from build123d import *

# Parameters (mm, degrees)
EXTRUDE_THIN1_DEPTH      = 28
EXTRUDE_THIN1_DEPTH_BACK = 8


with BuildPart() as part:
    # Sketch1 → Extrude-Thin1 (new, two sides: drawn at the far end of the back side and taken through both)
    with BuildSketch(Plane.XY.offset(-EXTRUDE_THIN1_DEPTH_BACK)):
        with BuildLine():
            Line((19.383566169, -68.309294305), (57.022380557, -25.814786092))
            ThreePointArc((57.022380557, -25.814786092), (65.70728891, -19.214238602), (76.255341013, -16.4333292))
            Line((76.255341013, -16.4333292), (228.091165061, -7.048771065))
            ThreePointArc((228.091165061, -7.048771065), (323.514042398, -112.549255422), (199.474713255, -182.192076622))
            Line((199.474713255, -182.192076622), (-76.082369589, -70.323577063))
            ThreePointArc((-76.082369589, -70.323577063), (-86.509762237, -25.814215154), (-41.067256055, -30.793416585))
            Line((-41.067256055, -30.793416585), (-22.813516306, -63.686280276))
            ThreePointArc((-22.813516306, -63.686280276), (-2.911096467, -76.915520396), (19.383566169, -68.309294305))
        make_face()
        with BuildLine():
            Line((26.869376151, -74.939727844), (64.508190539, -32.44521963))
            ThreePointArc((64.508190539, -32.44521963), (70.091345909, -28.20201053), (76.872236546, -26.414283057))
            Line((76.872236546, -26.414283057), (228.708060595, -17.029724922))
            ThreePointArc((228.708060595, -17.029724922), (313.644907456, -110.93674946), (203.236273822, -172.926513385))
            Line((203.236273822, -172.926513385), (-72.320809021, -61.058013827))
            ThreePointArc((-72.320809021, -61.058013827), (-79.024132867, -32.444852599), (-49.811093178, -35.645767804))
            Line((-49.811093178, -35.645767804), (-31.557353429, -68.538631496))
            ThreePointArc((-31.557353429, -68.538631496), (-4.00015673, -86.856040893), (26.869376151, -74.939727844))
        make_face(mode=Mode.SUBTRACT)
    extrude(amount=EXTRUDE_THIN1_DEPTH + EXTRUDE_THIN1_DEPTH_BACK)


solid = part.part
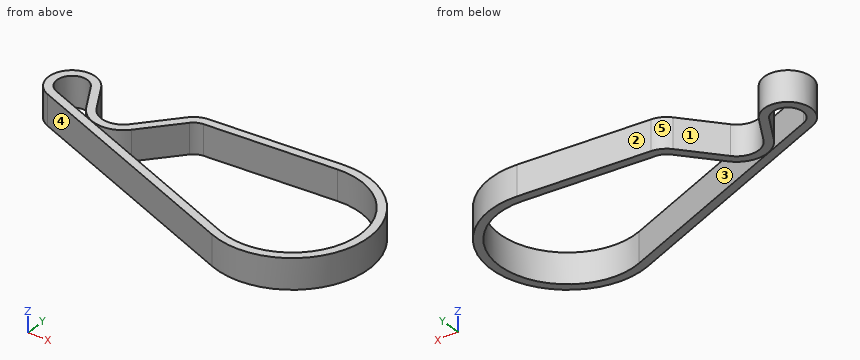
Read the model definition and answer for the solid it produces. Units are mm, in the model's axes. Face numbers are marked on the shaded views. A direction names the side the tool comes from. Round coordinates to 2 decimals unless told otherwise and drop trailing zeros. Loops run counter-clockwise (first coordinate to the right, second up) from the corner with the lowest first, then second, coordinate; pieces in that order, holes last.
Q1. Section C-C on y = -44.38 is taken. Write down the section's boundary in (x, z), and give its area (3 significant figures).
Q2. Section A-A on z = 2.5 is taken. Write down the section's boundary in (x, y).
Q3. Determine the mould class of the marked faces 1 and 2 for opening direction X: released by +X, released by -X, zero draft, split by the parting line, or undercut.
Q4. Consider probe 1 along X at (y, z) = (-70, -4.5); probe 2 along X at (y, z) = (-52, -1); probe 3 along Y at (x, z) = (258, -5.5). Determine where each line is inside the solid, lowest interval first.
Q5. Section D-D on x = 254.5 is taken. Write down the section's boundary in (y, z), and give its area (3 significant figures).
Q6. Section B-B on x = 68.5 is taken. Write down the section's boundary in (y, z), and give its area (3 significant figures).
Q7. Each of these flat-tipped pins is pushed along its axis until it touches: pin 1 (12 mm diameter, centred on y = -159, z = 14.5, fed in from +X); pin 2 (2 mm diameter, centred on x = 100.5, z = -1.5, fed in from -Y); pin 3 (5 mm diameter, centred on x = -1.5, z = 14.5, fed in from +Y). Where does it stop, or does it pass through?
Q8. Which of the six approach directions +Z, -Z, +X, -X, +Y, -Y give full straight-line access (tool end or side, diameter ignored) to the marked faces 3, 4 and 5?
Output:
1. outline: (-93.55, -8) - (-83.55, -8) - (-83.55, 28) - (-93.55, 28) - close; (-44.96, -8) - (-33.53, -8) - (-33.53, 28) - (-44.96, 28) - close; (40.58, -8) - (53.94, -8) - (53.94, 28) - (40.58, 28) - close; (294.53, -8) - (307.32, -8) - (307.32, 28) - (294.53, 28) - close
1. area: 1,710 mm2
2. outline: (-76.08, -70.32) - (199.47, -182.19) arc R91 ccw (long way) to (228.09, -7.05) - (76.26, -16.43) arc R28 ccw to (57.02, -25.81) - (19.38, -68.31) arc R26 cw to (-22.81, -63.69) - (-41.07, -30.79) arc R28 ccw (long way) to start; hole (-72.32, -61.06) - (203.24, -172.93) arc R81 ccw (long way) to (228.71, -17.03) - (76.87, -26.41) arc R18 ccw to (64.51, -32.45) - (26.87, -74.94) arc R36 cw to (-31.56, -68.54) - (-49.81, -35.65) arc R18 ccw (long way) to start
3. face 1: undercut
3. face 2: released by -X
4. probe 1: x = -76.85 to -50.29, -30.7 to -17.9, 17.74 to 31.24, 309.76 to 320.33
4. probe 2: x = -92.49 to -81.86, -40.74 to -29.3, 33.83 to 47.19, 300.46 to 312.3
4. probe 3: y = -185.57 to -175.15, -20.6 to -10.18
5. outline: (-186.47, -8) - (-176.16, -8) - (-176.16, 28) - (-186.47, 28) - close; (-19.59, -8) - (-9.28, -8) - (-9.28, 28) - (-19.59, 28) - close
5. area: 742 mm2
6. outline: (-129.02, -8) - (-118.23, -8) - (-118.23, 28) - (-129.02, 28) - close; (-29.08, -8) - (-18.03, -8) - (-18.03, 28) - (-29.08, 28) - close
6. area: 786 mm2
7. pin 1: stops at x = 306.11
7. pin 2: stops at y = -142.42
7. pin 3: stops at y = -76.77
8. face 3: +Z, -Z
8. face 4: +Z, -Z, -X, -Y
8. face 5: +Z, -Z, +Y
